```python
from build123d import *

# Parameters (mm, degrees)
F1_DEPTH    = 9.525
F2_R        = 1.5875
F3_DEPTH    = 12.701
F4_T1_DEPTH = 21.336
F4_T3_DEPTH = 16.266474116


# Not quite as in the source:
# - a fillet or chamfer that OpenCascade refuses, or shapes differently, is made with other operations: its cross-section is extruded or revolved along the edge and cut away or added


with BuildPart() as f1:
    # F0 (on Top) → F1 (new body)
    with BuildSketch(Plane.XY):
        with BuildLine():
            Line((24.2244322948, 0), (0, 0))
            Line((0, 0), (0, -3.175))
            Line((0, -3.175), (31.75, -3.175))
            Line((31.75, -3.175), (31.75, 0))
            Line((31.75, 0), (25.748250134, 1.5004374665))
            ThreePointArc((25.748250134, 1.5004374665), (25.2936999645, 0.4380706052), (24.2244322948, 0))
        make_face()
        with BuildLine():
            ThreePointArc((24.9994406757, 2.8362263561), (25.5538056385, 2.2692130656), (25.748250134, 1.5004374665))
            Line((25.748250134, 1.5004374665), (31.75, 0))
            ThreePointArc((31.75, 0), (28.9601920908, 6.7351920908), (22.225, 9.525))
            Line((22.225, 9.525), (19.05, 9.525))
            Line((19.05, 9.525), (19.05, 6.35))
            Line((19.05, 6.35), (24.9994406757, 2.8362263561))
        make_face()
    extrude(amount=F1_DEPTH)

    # F2 (on face) → F3 (cut, through all)
    with BuildSketch(Plane.XZ.offset(3.175)):
        with Locations((9.525, 4.7625)):
            Circle(F2_R)
    extrude(amount=-F3_DEPTH, mode=Mode.SUBTRACT)

    # F4: fillet of radius 2.3622 on 5 edges, made by hand

    # F4_s2 → F4_t1 (cut)
    with BuildSketch(Plane.XY.offset(-5.9055)):
        with BuildLine():
            ThreePointArc((29.3878, -3.175), (31.0581276385, -2.4831276385), (31.75, -0.8128))
            Line((31.75, -0.8128), (31.75, -3.175))
            Line((31.75, -3.175), (29.3878, -3.175))
        make_face()
        with BuildLine():
            ThreePointArc((21.4122, 9.525), (19.7418723615, 8.8331276385), (19.05, 7.1628))
            Line((19.05, 7.1628), (19.05, 9.525))
            Line((19.05, 9.525), (21.4122, 9.525))
        make_face()
        with BuildLine():
            ThreePointArc((0, -0.8128), (0.6918723615, -2.4831276385), (2.3622, -3.175))
            Line((2.3622, -3.175), (0, -3.175))
            Line((0, -3.175), (0, -0.8128))
        make_face()
        with BuildLine():
            ThreePointArc((2.3622, 0), (0.6918723615, -0.6918723615), (0, -2.3622))
            Line((0, -2.3622), (0, 0))
            Line((0, 0), (2.3622, 0))
        make_face()
    extrude(amount=F4_T1_DEPTH, mode=Mode.SUBTRACT)

    # F4_s4 → F4_t3 (cut)
    with BuildSketch(Plane.XY.offset(-3.370737058)):
        with BuildLine():
            ThreePointArc((20.2109370097, 5.6643439713), (19.3606624942, 6.5273197158), (19.05, 7.6982948232))
            Line((19.05, 7.6982948232), (19.05, 6.35))
            Line((19.05, 6.35), (20.2109370097, 5.6643439713))
        make_face()
    extrude(amount=F4_T3_DEPTH, mode=Mode.SUBTRACT)


solid = f1.part
```
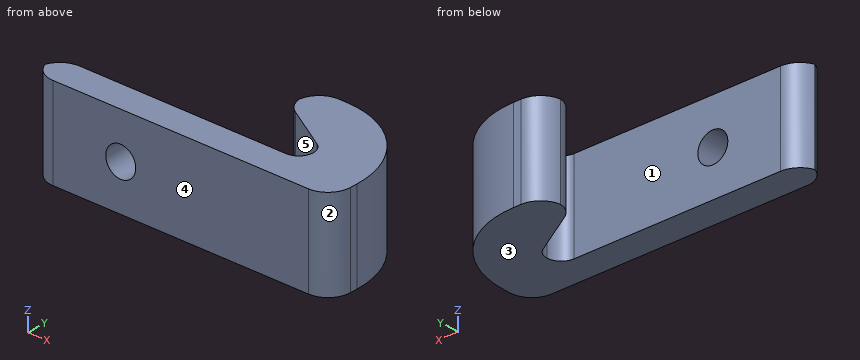
Build history of the part. All positions in model axes, mm. Face numbers are marked on the shaded views. A direction names the side the tool comes from. Give positions to 0.01 mm unless a question says otherwise; leave off trailing zeros. Loops run counter-clockwise (first coordinate to the right, second up) from the corner with the lowest first, then second, coordinate; pieces in that order, holes last.
Item 1: Which spindle directions (+Z, -Z, +X, -X, +Y, -Y) get a long thin tool onto all of the face, cutting with end or side? Do the marked faces 4 and 5. Say none if no direction does.
Answers follow:
face 4: +Z, -Z, +X, -X, -Y
face 5: +Z, -Z, -X
Item 2: Slice it at B-B, the plane x = 23.5. List the corners of the cut face in (y, z) (3 decimals), and give its area (3 significant figures).
Answers follow:
outline: (-3.175, 0) - (0, 0) - (0, 9.525) - (-3.175, 9.525) - close; (3.722, 0) - (9.439, 0) - (9.439, 9.525) - (3.722, 9.525) - close
area: 84.7 mm2
Item 3: Pull direction Y, two halves, no side cores. Call the marked faces 1, 2 and 3: released by +Y, released by -Y, zero draft, split by the parting line, or undercut.
Answers follow:
face 1: undercut
face 2: released by -Y
face 3: zero draft
Item 4: Drill centre lines: line 1 (Y direction, x = 4.5, z = 5.5) (3 decimals); line 2 (Y direction, x = 22, z = 3) (3 decimals); line 3 (Y direction, x = 22.5, z = 6.25) (3 decimals). Where is each one in solid material? Low to high.
Answers follow:
line 1: y = -3.175 to 0
line 2: y = -3.175 to 0, 4.608 to 9.525
line 3: y = -3.175 to 0, 4.312 to 9.521
Item 5: Slice it at D-D, the plane x = 17. List the corners of the cut face in (y, z) (3 decimals).
Answers follow:
outline: (-3.175, 0) - (0, 0) - (0, 9.525) - (-3.175, 9.525) - close
Item 6: Flat gauge pins, fed straight in: pin 1 (4 mm diameter, centred on y = 5.5, z = 3, fed in from +X); pin 2 (3 mm diameter, centred on x = 10.5, z = 7, fed in from +Y); pin 3 (4 mm diameter, centred on y = 0.5, z = 2.5, fed in from -X). Where does each tip first touch, or does it go through?
Answers follow:
pin 1: stops at x = 31.08
pin 2: stops at y = 0
pin 3: stops at x = 0.16
